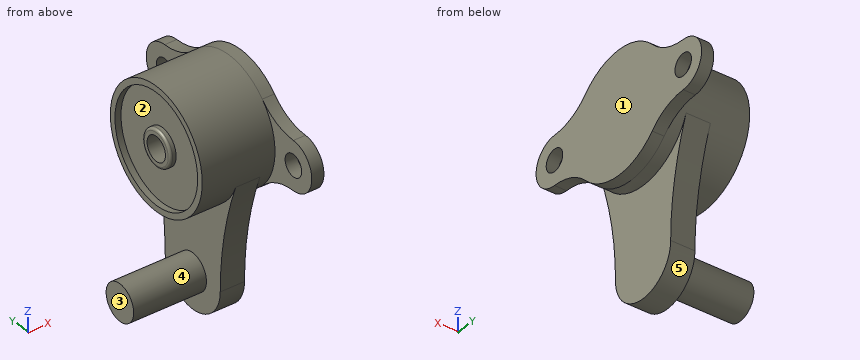
```python
from build123d import *
from build123d.topology import SkipClean

# Parameters (mm, degrees)
FILLET1_R           = 1
SKETCH2_R           = 4.5
BOSS_EXTRUDE2_DEPTH = 5
BOSS_EXTRUDE3_DEPTH = 10
SKETCH4_R           = 7.5
BOSS_EXTRUDE4_DEPTH = 30


with BuildPart() as part:
    # Sketch1 → Revolve1 (revolve)
    with BuildSketch(Plane.XY, mode=Mode.PRIVATE) as revolve1_sk:
        Polygon((15, 25), (-15, 25), (-15, 22.5), (-12.5, 22.5), (-12.5, 7.5), (-15, 7.5), (-15, 5), (15, 5), align=None)
    revolve(revolve1_sk.sketch.rotate(Axis((0, 0, 0), (-1, 0, 0)), 90), axis=Axis((0, 0, 0), (-1, 0, 0)))

    # Fillet1
    fillet1_edges = [part.edges().sort_by_distance(p)[0] for p in [
        (-15, 0, 7.5),
    ]]
    fillet(fillet1_edges, radius=FILLET1_R)

    # Sketch2 → Boss-Extrude2 (add)
    with SkipClean():  # the faces are left unmerged after this step: merging them gives an invalid solid
        with BuildSketch(Plane(origin=(15, 0, 0), x_dir=(0, 0, -1), z_dir=(1, 0, 0))):
            with BuildLine():
                ThreePointArc((10, 35), (0, 45), (-10, 35))
                ThreePointArc((-10, 35), (-11.886615966, 25.8085497), (-17.24137931, 18.103448276))
                ThreePointArc((-17.24137931, 18.103448276), (-25, 0), (-17.24137931, -18.103448276))
                ThreePointArc((-17.24137931, -18.103448276), (-11.886615966, -25.8085497), (-10, -35))
                ThreePointArc((-10, -35), (0, -45), (10, -35))
                ThreePointArc((10, -35), (11.886615966, -25.8085497), (17.24137931, -18.103448276))
                ThreePointArc((17.24137931, -18.103448276), (25, 0), (17.24137931, 18.103448276))
                ThreePointArc((17.24137931, 18.103448276), (11.886615966, 25.8085497), (10, 35))
            make_face()
            with Locations((0, 35)):
                Circle(SKETCH2_R, mode=Mode.SUBTRACT)
            with Locations((0, -35)):
                Circle(SKETCH2_R, mode=Mode.SUBTRACT)
        extrude(amount=BOSS_EXTRUDE2_DEPTH)

    # Sketch3 → Boss-Extrude3 (add)
    with SkipClean():  # the faces are left unmerged after this step: merging them gives an invalid solid
        with BuildSketch(Plane(origin=(0, 0, 0), x_dir=(0, 0, -1), z_dir=(1, 0, 0))):
            with BuildLine():
                Line((8.8, 23.4), (8.8, -23.4))
                ThreePointArc((8.8, -23.4), (31.521286236, -17.117074299), (55, -15))
                ThreePointArc((55, -15), (70, 0), (55, 15))
                ThreePointArc((55, 15), (31.521286236, 17.117074299), (8.8, 23.4))
            make_face()
        extrude(amount=BOSS_EXTRUDE3_DEPTH)

    # Sketch4 → Boss-Extrude4 (add)
    with SkipClean():  # the faces are left unmerged after this step: merging them gives an invalid solid
        with BuildSketch(Plane.ZY):
            with Locations((-55, 0)):
                Circle(SKETCH4_R)
        extrude(amount=BOSS_EXTRUDE4_DEPTH)


solid = part.part
```
Part model, mm, in its own coordinate system. Face numbers are marked on the shaded views. A direction names the side the tool comes from. Round coordinates to 2 decimals unless told otherwise and drop trailing zeros. Write each loop counter-clockwise with the first axis right and the second up, starting at its lowest first coordinate (ties: lowest second). Pieces come first, ordered by that corner, then holes.
Item 1: Cut at B-B, the plane x = 4.5. Give the cut face in (y, z).
Results:
outline: (-23.4, -8.8) arc R131.25 cw to (-15, -55) arc R15 ccw to (15, -55) arc R131.25 cw to (23.4, -8.8) arc R25 ccw (long way) to start; hole circle Ø10 at (0, 0)
Item 2: Which spindle directions (+Z, -Z, +X, -X, +Y, -Y) get a long thin tool onto all of the face, cutting with end or side? Do the marked faces 1 and 2. Say none if no direction does.
Results:
face 1: +Z, -Z, +X, +Y, -Y
face 2: -X
Item 3: Probe L1, parallel to Y at x = -13, z = 0; L2, parallel to Y at x = 18.1, z = 0; L3, parallel to Y at x = 1, z = 0. List the from-to ranges inside material, lowest first.
Results:
L1: y = -25 to -22.5, -7.5 to -5, 5 to 7.5, 22.5 to 25
L2: y = -45 to -39.5, -30.5 to 30.5, 39.5 to 45
L3: y = -25 to -5, 5 to 25
Item 4: Cut at A-A, the plane z = 0. Count the separate pieces of the cut face and the enclosed holes in it, plus the area to 3 significant figures.
Results:
separate pieces: 3
enclosed holes: 0
area: 1,480 mm2
Item 5: Two-plate mould, pull along Z, no slides. Class the marked faces 3, 4 and 5: +Z half, -Z half, draft (parallel to the pull), parting line (faces both ways), or undercut.
Results:
face 3: draft
face 4: undercut
face 5: -Z half
Item 6: Cut at D-D, the plane z = -58.5. Give the cut face in (x, y), plus the area to 3 significant figures.
Results:
outline: (-30, -6.63) - (0, -6.63) - (0, -14.59) - (10, -14.59) - (10, 14.59) - (0, 14.59) - (0, 6.63) - (-30, 6.63) - close
area: 690 mm2
Item 7: Cut at C-C, the plane y = -32.5. Give the cut face in (x, z), plus the area to 3 significant figures.
Results:
outline: (15, -10.13) - (20, -10.13) - (20, -3.74) - (15, -3.74) - close; (15, 3.74) - (20, 3.74) - (20, 10.13) - (15, 10.13) - close
area: 63.9 mm2
Item 8: Drop flat-ended pins along their axis: pin 1 Ø5 at (x, z) = (-7.5, -17) entering from -Y; pin 2 Ø10 at (y, z) = (-2.5, -19.5) entering from -X; pin 3 Ø2 at (x, z) = (-14.5, -2) entering from -Y; pin 4 Ø1 at (x, z) = (-2, -35) entering from -Y. Give the stop position or say it passes through.
Results:
pin 1: stops at y = -20.37
pin 2: stops at x = -15
pin 3: stops at y = -24.98
pin 4: passes through
